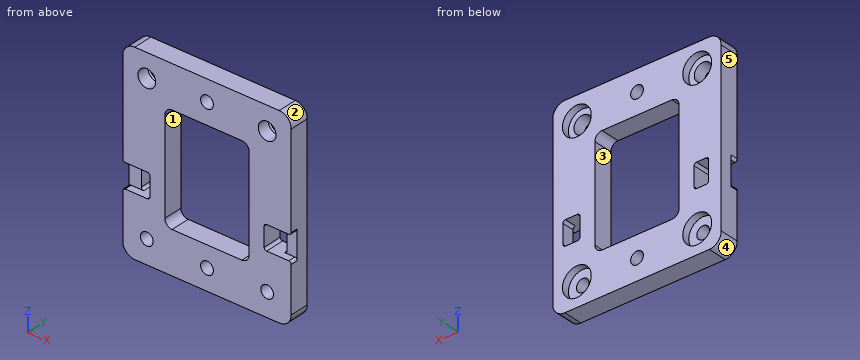
from build123d import *

# Parameters (mm, degrees)
CROQUIS1_R              = 2.65
CROQUIS1_R_2            = 6
SALIENTE_EXTRUIR1_DEPTH = 8
CROQUIS1_4_R            = 6
CROQUIS1_4_R_2          = 3.7
CROQUIS1_4_R_3          = 2.65
SALIENTE_EXTRUIR2_DEPTH = 5
CROQUIS1_6_R            = 3.7
CROQUIS1_6_R_2          = 2.65
CORTAR_EXTRUIR1_DEPTH   = 5
CORTAR_EXTRUIR2_DEPTH   = 3


with BuildPart() as part:
    # Croquis1 → Saliente-Extruir1 (new body)
    with BuildSketch(Plane(origin=(0, 0, 0), x_dir=(1, 0, 0), z_dir=(0, 1, 0))):
        with BuildLine():
            Line((-35, -35), (-35, 35))
            ThreePointArc((-35, 35), (-33.535533906, 38.535533906), (-30, 40))
            Line((-30, 40), (30, 40))
            ThreePointArc((30, 40), (33.535533906, 38.535533906), (35, 35))
            Line((35, 35), (35, -35))
            ThreePointArc((35, -35), (33.535533906, -38.535533906), (30, -40))
            Line((30, -40), (-30, -40))
            ThreePointArc((-30, -40), (-33.535533906, -38.535533906), (-35, -35))
        make_face()
        with Locations((0, 31.2526)):
            Circle(CROQUIS1_R, mode=Mode.SUBTRACT)
        with Locations((0, -31.2526)):
            Circle(CROQUIS1_R, mode=Mode.SUBTRACT)
        with Locations((-24.99964, -30.24738)):
            Circle(CROQUIS1_R_2, mode=Mode.SUBTRACT)
        with Locations((-24.99964, 30.25392)):
            Circle(CROQUIS1_R_2, mode=Mode.SUBTRACT)
        with Locations((24.99964, -30.24738)):
            Circle(CROQUIS1_R_2, mode=Mode.SUBTRACT)
        with Locations((24.99964, 30.25392)):
            Circle(CROQUIS1_R_2, mode=Mode.SUBTRACT)
        with BuildLine():
            Line((-14.5, -22.5), (14.5, -22.5))
            ThreePointArc((14.5, -22.5), (16.621320344, -21.621320344), (17.5, -19.5))
            Line((17.5, -19.5), (17.5, 19.5))
            ThreePointArc((17.5, 19.5), (16.621320344, 21.621320344), (14.5, 22.5))
            Line((14.5, 22.5), (-14.5, 22.5))
            ThreePointArc((-14.5, 22.5), (-16.621320344, 21.621320344), (-17.5, 19.5))
            Line((-17.5, 19.5), (-17.5, -19.5))
            ThreePointArc((-17.5, -19.5), (-16.621320344, -21.621320344), (-14.5, -22.5))
        make_face(mode=Mode.SUBTRACT)
        with BuildLine():
            Line((24.75, 15), (29.75, 15))
            ThreePointArc((29.75, 15), (30.457106781, 14.707106781), (30.75, 14))
            Line((30.75, 14), (30.75, 6))
            ThreePointArc((30.75, 6), (30.457106781, 5.292893219), (29.75, 5))
            Line((29.75, 5), (24.75, 5))
            ThreePointArc((24.75, 5), (24.042893219, 5.292893219), (23.75, 6))
            Line((23.75, 6), (23.75, 14))
            ThreePointArc((23.75, 14), (24.042893219, 14.707106781), (24.75, 15))
        make_face(mode=Mode.SUBTRACT)
        with BuildLine():
            Line((-28.75, 15), (-24.75, 15))
            ThreePointArc((-24.75, 15), (-24.042893219, 14.707106781), (-23.75, 14))
            Line((-23.75, 14), (-23.75, 6))
            ThreePointArc((-23.75, 6), (-24.042893219, 5.292893219), (-24.75, 5))
            Line((-24.75, 5), (-28.75, 5))
            ThreePointArc((-28.75, 5), (-29.457106781, 5.292893219), (-29.75, 6))
            Line((-29.75, 6), (-29.75, 14))
            ThreePointArc((-29.75, 14), (-29.457106781, 14.707106781), (-28.75, 15))
        make_face(mode=Mode.SUBTRACT)
    extrude(amount=SALIENTE_EXTRUIR1_DEPTH)

    # Croquis1_4 → Saliente-Extruir2 (add)
    with BuildSketch(Plane(origin=(0, 0, 0), x_dir=(1, 0, 0), z_dir=(0, 1, 0))):
        with Locations((-24.99964, -30.24738)):
            Circle(CROQUIS1_4_R)
        with Locations((-24.99964, -30.24738)):
            Circle(CROQUIS1_4_R_2, mode=Mode.SUBTRACT)
        with Locations((-24.99964, 30.25392)):
            Circle(CROQUIS1_4_R)
        with Locations((-24.99964, 30.25392)):
            Circle(CROQUIS1_4_R_3, mode=Mode.SUBTRACT)
        with Locations((24.99964, 30.25392)):
            Circle(CROQUIS1_4_R)
        with Locations((24.99964, -30.24738)):
            Circle(CROQUIS1_4_R)
    extrude(amount=SALIENTE_EXTRUIR2_DEPTH)

    # Croquis1_6 → Cortar-Extruir1 (cut)
    with BuildSketch(Plane(origin=(0, 0, 0), x_dir=(1, 0, 0), z_dir=(0, 1, 0))):
        with Locations((24.99964, -30.24738)):
            Circle(CROQUIS1_6_R)
        with Locations((24.99964, 30.25392)):
            Circle(CROQUIS1_6_R_2)
    extrude(amount=CORTAR_EXTRUIR1_DEPTH, mode=Mode.SUBTRACT)

    # Croquis3 → Cortar-Extruir2 (cut)
    with BuildSketch(Plane.XZ):
        with BuildLine():
            Line((-35, -4), (-35, -16))
            ThreePointArc((-35, -16), (-34.707106781, -15.292893219), (-34, -15))
            Line((-34, -15), (-28.75, -15))
            Line((-28.75, -15), (-28.75, -5))
            Line((-28.75, -5), (-34, -5))
            ThreePointArc((-34, -5), (-34.707106781, -4.707106781), (-35, -4))
        make_face()
        with BuildLine():
            Line((35, -4), (35, -16))
            ThreePointArc((35, -16), (34.707106781, -15.292893219), (34, -15))
            Line((34, -15), (29.75, -15))
            Line((29.75, -15), (29.75, -5))
            Line((29.75, -5), (34, -5))
            ThreePointArc((34, -5), (34.707106781, -4.707106781), (35, -4))
        make_face()
    extrude(amount=-CORTAR_EXTRUIR2_DEPTH, mode=Mode.SUBTRACT)


solid = part.part
Geometry check sheet. Reference: the model listing, model coordinates, mm. Face numbers are marked on the shaded views. A direction names the side the tool comes from. Coordinates: 2 decimals unless noted, no trailing zeros. Order: outer loops, then holes, each group sorted by start corner. A loop starts at its lowest first (then second) coordinate and runs counter-clockwise, first axis right, second up. Notation, with made-up numbers: (57, -1.5) -> (114, -1.5) arc R31 ccw to (114, 34.5) -> close; hole circle Ø6 at (36.5, 63.25). An arc over 180 degrees is marked (long way). Use a Markdown table: item, result. Add a question column.
1. Cross-section at B-B (z = 1.5). Enter the section's corners in (x, y), and give its area (3 significant figures).
2. Cross-section at D-D (y = 1.75). Give the number of separate pieces and of enclosed holes in the cut face, and give its area (3 significant figures).
3. Cross-section at A-A (x = 0). Enter the section's corners in (y, z), and give its area (3 significant figures).
4. Mould release check, pull along Z, two halves, no side actions. Record for the marked faces 3, 4 and 5: pulls with the +Z half, pulls with the -Z half, needs draft (parallel to the pull), parting line crosses it, or undercut.
5. Material ranges on L1, parallel to Z at x = 0, y = 4; L2, parallel to X at y = 3.25, z = -11.5; L3, parallel to Z at x = 4, y = 3.25, recorded low to high.
6. Go/stop test with flat-tipped pins: pin 1 Ø1.9 at (x, z) = (-33, -10.5) entering from -Y; pin 2 Ø3.5 at (x, z) = (-23, 33) entering from +Y; pin 3 Ø14 at (x, z) = (-25, -30.25) entering from -Y. Record where each tip stops, or that it passes through.
7. Set-up check for the marked faces 1 and 2: record each of +Z, -Z, +X, -X, +Y, -Y from which the full face is reachable in a straight line by a thin tool's end or side.
8. Cross-section at C-C (x = -10). Enter the section's corners in (y, z), and give its area (3 significant figures).
Filled sheet:
| question | item | result |
|---|---|---|
| 1 | outline | (-35, 0) -> (-17.5, 0) -> (-17.5, 8) -> (-35, 8) -> close; (17.5, 0) -> (35, 0) -> (35, 8) -> (17.5, 8) -> close |
| 1 | area | 280 mm2 |
| 2 | separate pieces | 1 |
| 2 | enclosed holes | 7 |
| 2 | area | 3,610 mm2 |
| 3 | outline | (0, -40) -> (8, -40) -> (8, -33.9) -> (0, -33.9) -> close; (0, -28.6) -> (8, -28.6) -> (8, -22.5) -> (0, -22.5) -> close; (0, 22.5) -> (8, 22.5) -> (8, 28.6) -> (0, 28.6) -> close; (0, 33.9) -> (8, 33.9) -> (8, 40) -> (0, 40) -> close |
| 3 | area | 195 mm2 |
| 4 | face 3 | undercut |
| 4 | face 4 | pulls with the -Z half |
| 4 | face 5 | needs draft |
| 5 | L1 | -40 to -33.9, -28.6 to -22.5, 22.5 to 28.6, 33.9 to 40 |
| 5 | L2 | -35 to -29.75, -23.75 to -17.5, 17.5 to 23.75, 30.75 to 35 |
| 5 | L3 | -40 to -22.5, 22.5 to 40 |
| 6 | pin 1 | y = 3 |
| 6 | pin 2 | y = 5 |
| 6 | pin 3 | y = 0 |
| 7 | face 1 | +Y, -Y |
| 7 | face 2 | +Z, +X, +Y, -Y |
| 8 | outline | (0, -40) -> (8, -40) -> (8, -22.5) -> (0, -22.5) -> close; (0, 22.5) -> (8, 22.5) -> (8, 40) -> (0, 40) -> close |
| 8 | area | 280 mm2 |
